Check sheet for the modelled part. Datum: model origin and axes. Units: mm. Face numbers are marked on the shaded views. A direction names the side the tool comes from. Round coordinates to 2 decimals unless told otherwise and drop trailing zeros. Order: outer loops, then holes, each group sorted by start corner. A loop starts at its lowest first (then second) coordinate and runs counter-clockwise, first axis right, second up.
(1) Sectioned sample at B-B, the plane x = 30. Enter the section's corners in (y, z).
(2) Thickness scan on probe 1 along X at (y, z) = (15, 13); probe 2 along Z at (x, y) = (-8, -13.5); probe 3 along Y at (x, z) = (-13.25, 0). Record the ranges inside material, lowest first.
(3) Depth check by flat-ended pin: pin 1 (11.5 mm diameter, centred on y = 15.5, z = 8.5, fed in from +X); pin 2 (1.5 mm diameter, centred on y = -8, z = 15.5, fed in from -X); pin 3 (2.5 mm diameter, centred on x = 42, z = 11.5, fed in from +Y). Enter the tip coordinate at first touch or a pass-through.
(4) Sectioned sample at A-A, the plane x = 15.5. Enter the section's corners in (y, z).
(5) Tool access check on the marked faces 1, 2, 3 and 4. Record the directions out of +Z, -Z, +X, -X, +Y, -Y that give a thin tool (end or side, any length) a straight path to the whole face; none if there is none.
```python
from build123d import *

# Parameters (mm, degrees)
F3_DEPTH  = 5
F6_W      = 39
F6_H      = 21.8819705509
F6_H_2    = 21.9819051884
F7_DEPTH  = 18.6505033058
F8_W      = 39
F8_H      = 30.9849461095
F8_H_2    = 27.3872321026
F9_DEPTH  = 18.6505033058
F11_D     = 6
F11_DEPTH = 10
F11_TIP   = 1.8025818571
F12_SIZE  = 0.2
F13_R     = 8


with BuildPart() as f1:
    # F0 (on Front) → F1 (revolve)
    with BuildSketch(Plane.XZ):
        Polygon((-29.0833324906, 7.475), (-29.0833324906, 0), (43.9166675094, 0), (43.9166675094, 23), (-16.0833324906, 23), (-16.0833324906, 7.475), align=None)
    revolve(axis=Axis((6.4323022962, 0, 0), (1, 0, 0)))

    # F2 (on face) → F3 (cut)
    with BuildSketch(Plane.YZ.offset(43.9166675094)):
        with BuildLine():
            Line((-3, -22.803508502), (-3, 22.803508502))
            ThreePointArc((-3, 22.803508502), (-23, 0), (-3, -22.803508502))
        make_face()
        with BuildLine():
            ThreePointArc((23, 0), (17.2916164658, 15.1657508881), (3, 22.803508502))
            Line((3, 22.803508502), (3, -22.803508502))
            ThreePointArc((3, -22.803508502), (17.2916164658, -15.1657508881), (23, 0))
        make_face()
    extrude(amount=-F3_DEPTH, mode=Mode.SUBTRACT)

    # F6 (on offset) → F7 (cut, through all)
    with BuildSketch(Plane.XY.offset(4)):
        with Locations((11.4166675094, 14.9409852754)):
            Rectangle(F6_W, F6_H)
        with Locations((11.4166675094, -14.9909525942)):
            Rectangle(F6_W, F6_H_2)
    extrude(amount=F7_DEPTH, mode=Mode.SUBTRACT)

    # F8 (on offset) → F9 (cut, through all)
    with BuildSketch(Plane.XY.offset(-4)):
        with Locations((11.4166675094, -19.4924730548)):
            Rectangle(F8_W, F8_H)
        with Locations((11.4166675094, 17.6936160513)):
            Rectangle(F8_W, F8_H_2)
    extrude(amount=-F9_DEPTH, mode=Mode.SUBTRACT)

    # F11
    with Locations(Plane(origin=(-16.0833324906, 0, 0), x_dir=(0, -1, 0), z_dir=(-1, 0, 0))):
        with Locations((13.5, 0)):
            Hole(F11_D / 2, depth=F11_DEPTH)
            with Locations((0, 0, -(F11_DEPTH + F11_TIP / 2))):  # 118° drill point
                Cone(0, F11_D / 2, F11_TIP, mode=Mode.SUBTRACT)

    # F12
    f12_edges = [f1.edges().sort_by_distance(p)[0] for p in [
        (-16.083332, 0, -23),
        (38.916668, 23, 0),
        (38.916668, -23, 0),
        (43.916668, 1.503214, 22.950825),
        (43.916668, 0, -23),
        (43.916668, -1.503214, 22.950825),
        (-29.083332, 0, -7.475),
    ]]
    chamfer(f12_edges, length=F12_SIZE)

    # F13
    f13_edges = [f1.edges().sort_by_distance(p)[0] for p in [
        (-8.083332, -4, 13.324752),
        (30.916668, -4, 13.324752),
        (30.916668, 4, 13.324752),
        (-8.083332, 4, 13.324752),
        (-8.083332, -4, -13.324752),
        (30.916668, -4, -13.324752),
        (-8.083332, 4, -13.324752),
        (30.916668, 4, -13.324752),
    ]]
    fillet(f13_edges, radius=F13_R)


solid = f1.part
```
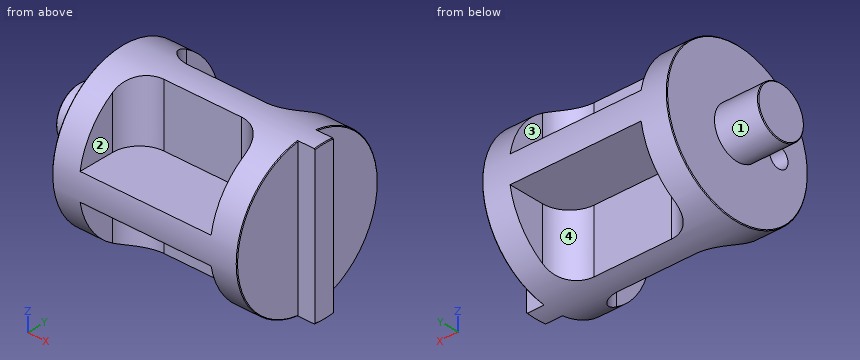
Derived:
1. outline: (-22.65, -4) - (-8.28, -4) - (-8.28, -21.46) arc R23 ccw to (8.28, -21.46) - (8.28, -4) - (22.65, -4) arc R23 ccw to (22.65, 4) - (8.28, 4) - (8.28, 21.46) arc R23 ccw to (-8.28, 21.46) - (-8.28, 4) - (-22.65, 4) arc R23 ccw to start
2. probe 1: x = -16.08 to -8.08, 30.92 to 38.92
2. probe 2: z = -4 to -3, 3 to 4
2. probe 3: y = -23 to -16.5, -10.5 to 23
3. pin 1: stops at x = 38.92
3. pin 2: stops at x = -16.08
3. pin 3: stops at y = 3
4. outline: (-22.65, -4) - (-4, -4) - (-4, -22.65) arc R23 ccw to (4, -22.65) - (4, -4) - (22.65, -4) arc R23 ccw to (22.65, 4) - (4, 4) - (4, 22.65) arc R23 ccw to (-4, 22.65) - (-4, 4) - (-22.65, 4) arc R23 ccw to start
5. face 1: -X
5. face 2: +Z, -Y
5. face 3: +Z, +Y
5. face 4: -Z, +Y
